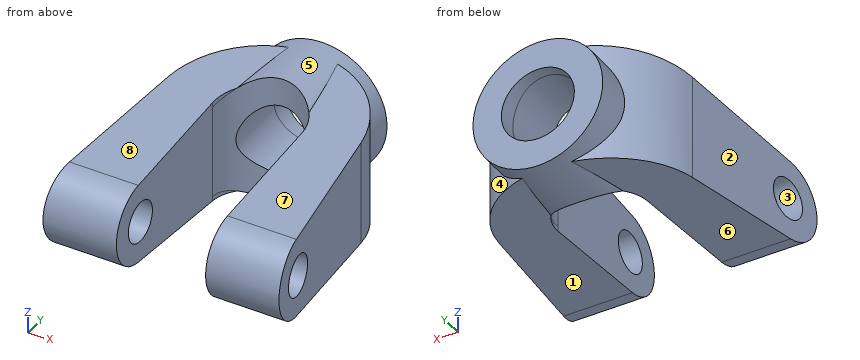
```python
from build123d import *

# Parameters (mm, degrees)
BOSS_EXTRUDE2_DEPTH     = 20
CUT_EXTRUDE5_DEPTH      = 74.091191345
CUT_EXTRUDE5_DEPTH_BACK = 74.091191345
SKETCH3_OUTSIDE_W       = 61.06
SKETCH3_OUTSIDE_H       = 85.06
SKETCH3_OUTSIDE_R       = 5
BOSS_EXTRUDE3_START     = 40
SKETCH4_R               = 16
SKETCH4_R_2             = 9
BOSS_EXTRUDE3_DEPTH     = 27
SKETCH4_4_R             = 9
CUT_EXTRUDE7_DEPTH      = 70
CUT_EXTRUDE8_DEPTH      = 75.775144726
CUT_EXTRUDE8_DEPTH_BACK = 75.775144726


with BuildPart() as part:
    # Sketch1 → Boss-Extrude2 (new, symmetric)
    with BuildSketch(Plane.XY):
        with BuildLine():
            ThreePointArc((-11, 40), (0, 51), (11, 40))
            Line((11, 40), (11, 18.669270992))
            ThreePointArc((11, 18.669270992), (20.493901532, 27.510004003), (24, 40))
            ThreePointArc((24, 40), (23.955235162, 41.465164949), (23.821107639, 42.924864242))
            ThreePointArc((23.821107639, 42.924864242), (0, 64), (-23.821107639, 42.924864242))
            ThreePointArc((-23.821107639, 42.924864242), (-21.218172289, 28.784423121), (-11, 18.669270992))
            Line((-11, 18.669270992), (-11, 40))
        make_face()
        with BuildLine():
            ThreePointArc((24, 40), (20.493901532, 27.510004003), (11, 18.669270992))
            Line((11, 18.669270992), (11, 0))
            Line((11, 0), (29.091618247, 0))
            Line((29.091618247, 0), (23.821107639, 42.924864242))
            ThreePointArc((23.821107639, 42.924864242), (23.955235162, 41.465164949), (24, 40))
        make_face()
        with BuildLine():
            Line((-11, 0), (-11, 18.669270992))
            ThreePointArc((-11, 18.669270992), (-21.218172289, 28.784423121), (-23.821107639, 42.924864242))
            Line((-23.821107639, 42.924864242), (-29.091618247, 0))
            Line((-29.091618247, 0), (-11, 0))
        make_face()
    extrude(amount=BOSS_EXTRUDE2_DEPTH, both=True)

    # Sketch3 outside → Cut-Extrude5 (cut, two sides: drawn at the far end of the back side and taken through both)
    # profile 1 of 2: a face of its own
    with BuildSketch(Plane(origin=(0, 0, 0), x_dir=(0, 0, -1), z_dir=(1, 0, 0)).offset(-CUT_EXTRUDE5_DEPTH_BACK)):
        with Locations((0, 32)):
            Rectangle(SKETCH3_OUTSIDE_W, SKETCH3_OUTSIDE_H)
        with BuildLine():
            Line((-14.886153969, 64), (-9.959975113, 9.106190314))
            ThreePointArc((-9.959975113, 9.106190314), (0, 0), (9.959975113, 9.106190314))
            Line((9.959975113, 9.106190314), (14.886153969, 64))
            Line((14.886153969, 64), (-14.886153969, 64))
        make_face(mode=Mode.SUBTRACT)
    # profile 2 of 2: a face of its own
    with BuildSketch(Plane(origin=(0, 0, 0), x_dir=(0, 0, -1), z_dir=(1, 0, 0)).offset(-CUT_EXTRUDE5_DEPTH_BACK)):
        with Locations(Location((0, 10, 0), (0, 0, 90))):
            Circle(SKETCH3_OUTSIDE_R)
    extrude(amount=CUT_EXTRUDE5_DEPTH + CUT_EXTRUDE5_DEPTH_BACK, mode=Mode.SUBTRACT)

    # Sketch4 → Boss-Extrude3 (add)
    with BuildSketch(Plane(origin=(0, 0, 0), x_dir=(1, 0, 0), z_dir=(0, 1, 0)).offset(BOSS_EXTRUDE3_START)):
        with Locations(Location((0, 0, 0), (0, 0, 270))):
            Circle(SKETCH4_R)
        with Locations(Location((0, 0, 0), (0, 0, 270))):
            Circle(SKETCH4_R_2, mode=Mode.SUBTRACT)
    extrude(amount=BOSS_EXTRUDE3_DEPTH)

    # Sketch4<4> → Cut-Extrude7 (cut)
    with BuildSketch(Plane(origin=(0, 0, 0), x_dir=(1, 0, 0), z_dir=(0, 1, 0))):
        with Locations(Location((0, 0, 0), (0, 0, 270))):
            Circle(SKETCH4_4_R)
    extrude(amount=CUT_EXTRUDE7_DEPTH, mode=Mode.SUBTRACT)

    # Sketch5 → Cut-Extrude8 (cut, two sides: drawn at the far end of the back side and taken through both)
    with BuildSketch(Plane.XY.offset(-CUT_EXTRUDE8_DEPTH_BACK)):
        with BuildLine():
            Line((-11, 40), (11, 40))
            ThreePointArc((11, 40), (10.4539787, 43.422620245), (8.870121938, 46.505454388))
            ThreePointArc((8.870121938, 46.505454388), (-3.422620245, 50.4539787), (-11, 40))
        make_face()
    extrude(amount=CUT_EXTRUDE8_DEPTH + CUT_EXTRUDE8_DEPTH_BACK, mode=Mode.SUBTRACT)


solid = part.part
```
Geometry check sheet. Reference: the model listing, model coordinates, mm. Face numbers are marked on the shaded views. A direction names the side the tool comes from. Round coordinates to 2 decimals unless told otherwise and drop trailing zeros. Write each loop counter-clockwise with the first axis right and the second up, starting at its lowest first coordinate (ties: lowest second). Pieces come first, ordered by that corner, then holes. Notation, with made-up numbers: (-35, 13.5) - (11, 13.5) arc R11 ccw to (11, 31.5) - close; hole circle Ø7 at (-7, 77.25). An arc over 180 degrees is marked (long way). Write each question's results on one line, items separated by ' | '.
(1) Sectioned sample at D-D, the plane y = 60.5. Enter the section's corners in (x, z).
Computed:
outline: (-12.48, -14.57) - (-6.61, -14.57) arc R16 ccw to (6.61, -14.57) - (12.48, -14.57) - (12.48, -10.01) arc R16 ccw to (12.48, 10.01) - (12.48, 14.57) - (6.61, 14.57) arc R16 ccw to (-6.61, 14.57) - (-12.48, 14.57) - (-12.48, 10.01) arc R16 ccw to (-12.48, -10.01) - close; hole circle Ø18 at (0, 0)
(2) Set-up check for the marked faces 4, 5, 6, 7 and 8: record each of +Z, -Z, +X, -X, +Y, -Y from which the full face is reachable in a straight line by a thin tool's end or side.
Computed:
face 4: +X, +Y | face 5: none | face 6: -Z, -X, -Y | face 7: +Z, +X, -Y | face 8: +Z, -X, -Y
(3) Draft check along Y on the marked faces 1, 2 and 3. Enter one of: pulls with the +Y half, pulls with the -Y half, needs draft (parallel to the pull), parting line crosses it, or undercut.
Computed:
face 1: pulls with the -Y half | face 2: pulls with the +Y half | face 3: undercut
(4) Sectioned sample at A-A, the plane x = 0. Enter the section's corners in (y, z).
Computed:
outline: (51, -16) - (67, -16) - (67, -9) - (51, -9) - close; (51, 9) - (67, 9) - (67, 16) - (51, 16) - close
(5) Sectioned sample at B-B, the plane y = 18.5. Enter the section's corners in (x, z).
Computed:
outline: (-26.82, -10.8) - (-11, -10.8) - (-11, 10.8) - (-26.82, 10.8) - close; (11, -10.8) - (26.82, -10.8) - (26.82, 10.8) - (11, 10.8) - close
(6) Sectioned sample at C-C, the plane z = -6. Enter the section's corners in (x, y).
Computed:
outline: (-28.85, 2) - (-11, 2) - (-11, 40) arc R11 cw to (-6.71, 48.72) - (-6.71, 67) - (-14.83, 67) - (-14.83, 58.87) arc R24 ccw to (-23.82, 42.92) - close; (6.71, 48.72) arc R11 cw to (11, 40) - (11, 2) - (28.85, 2) - (23.82, 42.92) arc R24 ccw to (14.83, 58.87) - (14.83, 67) - (6.71, 67) - close
(7) Thickness scan on probe 1 along Y at (x, z) = (-15.25, 0); probe 2 along Z at (x, y) = (0, 63); probe 3 along Z at (x, y) = (-16, 10). Record the ranges inside material, lowest first. Write a range as from..to.
Computed:
probe 1: y = 0..5, 15..67 | probe 2: z = -16..-9, 9..16 | probe 3: z = -10.04..-5, 5..10.04
(8) Depth check by flat-ended pin: pin 1 Ø5 at (y, z) = (18, 1.5) entering from +X; pin 2 Ø2 at (y, z) = (46, -11.5) entering from +X; pin 3 Ø2 at (x, y) = (16.5, 13) entering from -Z. Enter the tip coordinate at first touch or a pass-through.
Computed:
pin 1: stops at x = 27.19 | pin 2: stops at x = 23.47 | pin 3: stops at z = -10.4
